Source: CAD feature listing. Evaluate the final solid. Frame: model axes, mm. Face numbers are marked on the shaded views. Give positions to 0.01 mm unless a question says otherwise; leave off trailing zeros. Order: outer loops, then holes, each group sorted by start corner. A loop starts at its lowest first (then second) coordinate and runs counter-clockwise, first axis right, second up.
from build123d import *

# Parameters (mm, degrees)
SKETCH1_R             = 14.6812
SKETCH1_R_2           = 11.5062
BEARING_EXTRUDE_DEPTH = 4.7625
BOSS_EXTRUDE2_DEPTH   = 3.175
FILLET1_R             = 2.54


with BuildPart() as part:
    # Sketch1 → Bearing extrude (new, symmetric)
    with BuildSketch(Plane(origin=(0, 0, 0), x_dir=(1, 0, 0), z_dir=(0, 1, 0))):
        with Locations(Location((0, 0, 0), (0, 0, 90))):
            Circle(SKETCH1_R)
        with Locations(Location((0, 0, 0), (0, 0, 90))):
            Circle(SKETCH1_R_2, mode=Mode.SUBTRACT)
    extrude(amount=BEARING_EXTRUDE_DEPTH, both=True)

    # Sketch1<5> → Boss-Extrude2 (add, symmetric)
    with BuildSketch(Plane(origin=(0, 0, 0), x_dir=(1, 0, 0), z_dir=(0, 1, 0))):
        with BuildLine():
            Line((-7.9375, -12.350454534), (-7.9375, -55.3212))
            Line((-7.9375, -55.3212), (7.9375, -55.3212))
            Line((7.9375, -55.3212), (7.9375, -99.7712))
            Line((7.9375, -99.7712), (44.936648924, -89.431503617))
            Line((44.936648924, -89.431503617), (21.89252839, -51.421360118))
            Line((21.89252839, -51.421360118), (28.680054014, -47.306338594))
            Line((28.680054014, -47.306338594), (35.467579639, -43.19131707))
            Line((35.467579639, -43.19131707), (13.190345938, -6.446115688))
            ThreePointArc((13.190345938, -6.446115688), (3.951379748, -14.13945655), (-7.9375, -12.350454534))
        make_face()
        with BuildLine():
            ThreePointArc((3.1115, -47.3837), (0, -50.4952), (-3.1115, -47.3837))
            Line((-3.1115, -47.3837), (-3.1115, -25.4127))
            ThreePointArc((-3.1115, -25.4127), (0, -22.3012), (3.1115, -25.4127))
            Line((3.1115, -25.4127), (3.1115, -47.3837))
        make_face(mode=Mode.SUBTRACT)
        with BuildLine():
            ThreePointArc((27.225742535, -38.905724532), (27.587064378, -41.259593312), (26.178120928, -43.179523014))
            ThreePointArc((26.178120928, -43.179523014), (23.824252147, -43.540844858), (21.904322445, -42.131901407))
            Line((21.904322445, -42.131901407), (10.513942867, -23.344030478))
            ThreePointArc((10.513942867, -23.344030478), (11.561564474, -19.070231995), (15.835362956, -20.117853603))
            Line((15.835362956, -20.117853603), (27.225742535, -38.905724532))
        make_face(mode=Mode.SUBTRACT)
    extrude(amount=BOSS_EXTRUDE2_DEPTH, both=True)

    # Fillet1
    fillet1_edges = [part.edges().sort_by_distance(p)[0] for p in [
        (13.190345938, 0, 6.446115688),
        (-7.9375, 0, 12.350454534),
    ]]
    fillet(fillet1_edges, radius=FILLET1_R)


solid = part.part
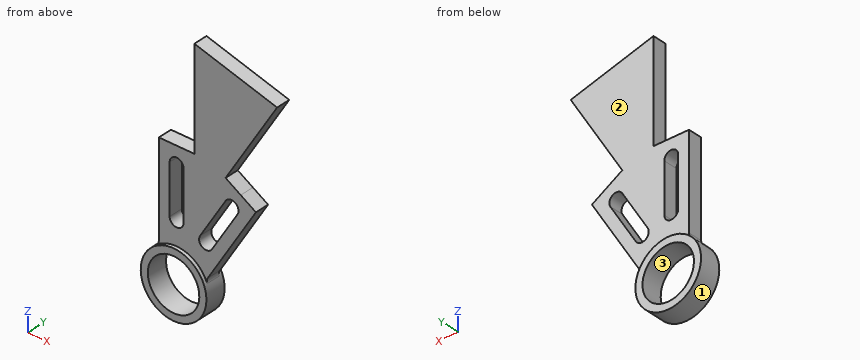
1) Section query C-C on y = -0.25. Output: boundary loops of the cut face in (x, z).
Checks:
outline: (-8.93, 11.65) arc R14.68 ccw (long way) to (13.68, 5.33) arc R2.54 cw to (13.87, 7.57) - (35.47, 43.19) - (21.89, 51.42) - (44.94, 89.43) - (7.94, 99.77) - (7.94, 55.32) - (-7.94, 55.32) - (-7.94, 13.67) arc R2.54 cw to start; hole circle Ø23.01 at (0, 0); hole (-3.11, 25.41) arc R3.11 ccw to (3.11, 25.41) - (3.11, 47.38) arc R3.11 ccw to (-3.11, 47.38) - close; hole (10.51, 23.34) arc R3.11 ccw to (15.84, 20.12) - (27.23, 38.91) arc R3.11 ccw to (21.9, 42.13) - close
2) Section query B-B on x = 0. Output: boundary loops of the cut face in (y, z) (1 decimal), and give its area (3 significant figures).
Checks:
outline: (-4.8, -14.7) - (4.8, -14.7) - (4.8, -11.5) - (-4.8, -11.5) - close; (-4.8, 11.5) - (4.8, 11.5) - (4.8, 14.7) - (3.2, 14.7) - (3.2, 22.3) - (-3.2, 22.3) - (-3.2, 14.7) - (-4.8, 14.7) - close; (-3.2, 50.5) - (3.2, 50.5) - (3.2, 55.3) - (-3.2, 55.3) - close
area: 140 mm2
3) Ray query, L1, parallel to X at y = -1.5, z = 0; L2, parallel to X at y = -1.5, z = 34; L3, parallel to Z at x = -1.5, y = 0.25. Return the intervals inside material, ascending.
Checks:
L1: x = -14.68 to -11.51, 11.51 to 14.68
L2: x = -7.94 to -3.11, 3.11 to 16.97, 24.25 to 29.9
L3: z = -14.6 to -11.41, 11.41 to 22.69, 50.11 to 55.32
4) Section query A-A on z = 0. Output: boundary loops of the cut face in (x, y), and give its area (3 significant figures).
Checks:
outline: (-14.68, -4.76) - (-11.51, -4.76) - (-11.51, 4.76) - (-14.68, 4.76) - close; (11.51, -4.76) - (14.68, -4.76) - (14.68, 4.76) - (11.51, 4.76) - close
area: 60.5 mm2
5) Section query D-D on z = 33. Output: boundary loops of the cut face in (x, y) (1 decimal), and give its area (3 significant figures).
Checks:
outline: (-7.9, -3.2) - (-3.1, -3.2) - (-3.1, 3.2) - (-7.9, 3.2) - close; (3.1, -3.2) - (16.4, -3.2) - (16.4, 3.2) - (3.1, 3.2) - close; (23.6, -3.2) - (29.3, -3.2) - (29.3, 3.2) - (23.6, 3.2) - close
area: 151 mm2
6) Pull-direction query (X, two-part tool) for the marked faces 1, 2 and 3; classes: +X half, -X half, draft (parallel to the pull), parting line (faces both ways), or undercut.
Checks:
face 1: parting line
face 2: draft
face 3: undercut
7) First-contact query: pin 1 Ø3 at (y, z) = (1.5, 34) entering from +X; pin 2 Ø8 at (x, z) = (26, 82.5) entering from +Y (3 decimals); pin 3 Ø12 at (x, z) = (0.5, -3) entering from -Y; pin 4 Ø1.5 at (x, z) = (11, 79) entering from -Y (3 decimals). Flat tips, straight axial feed; report the tip coordinate or a pass-through.
Checks:
pin 1: stops at x = 30.8
pin 2: stops at y = 3.175
pin 3: passes through
pin 4: stops at y = -3.175
